Check sheet for the drawn part. Datum: minimum x, y, z corner. Units: mm. Coordinates: 2 decimals unless noted, no trailing zeros. Loops run counter-clockwise (first coordinate to the right, second up) from the corner with the lowest first, then second, coordinate; pieces in that order, holes last. Notation, with made-up numbers: (56.5, -26) -> (70.5, -26) arc R14 ccw to (70.5, -4) -> close; hole circle Ø8 at (73, 67.25). An arc over 180 degrees is marked (long way). Use CSV: the item, a comma, the result in double quotes. Start each with the question number.
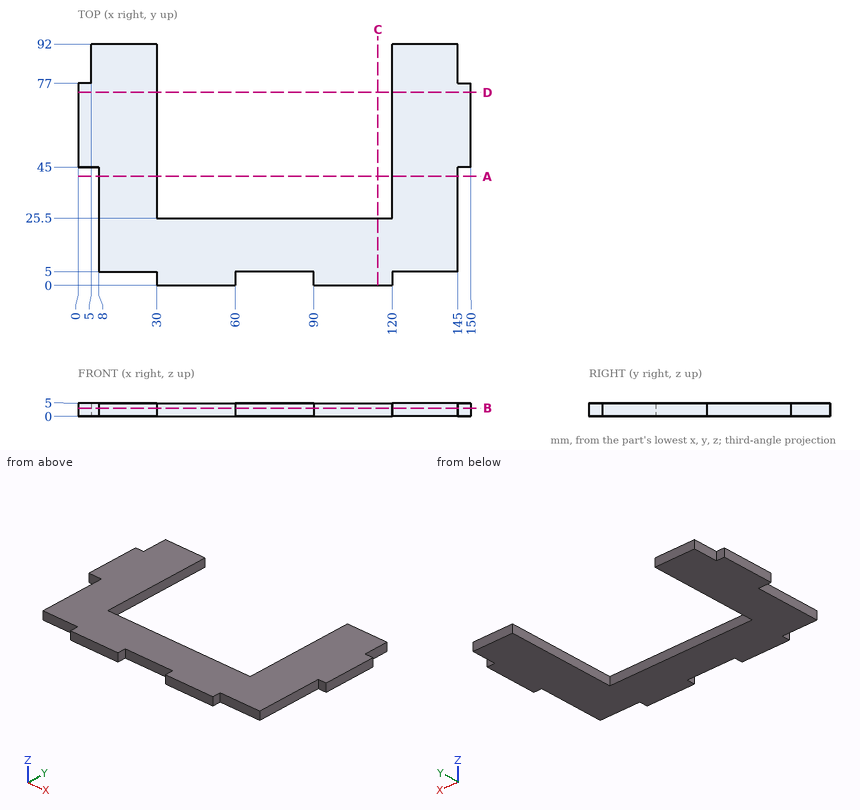
1. Cross-section at C-C, the plane x = 114.5. Record the boundary of the cut face in (y, z).
2. Cross-section at D-D, the plane y = 73.5. Record the boundary of the cut face in (x, z), plus the area to 3 significant figures.
3. Cross-section at A-A, the plane y = 41.5. Record the boundary of the cut face in (x, z).
4. Scan lines: line 1 (X direction, y = 29, z = 2.75); line 2 (X direction, y = 84.5, z = 4.55); line 3 (Y direction, x = 30.5, z = 2.9). Record each from-to range of solid material in increasing order.
5. Depth check by flat-ended pin: pin 1 (2.5 mm diameter, centred on x = 2, z = 1.5, fed in from -Y); pin 2 (2 mm diameter, centred on x = 123.5, z = 3, fed in from -Y); pin 3 (1.5 mm diameter, centred on y = 84.5, z = 1.5, fed in from -X). Enter the tip coordinate at first touch or a pass-through.
6. Cross-section at B-B, the plane z = 3.05. Record the boundary of the cut face in (x, y), plus the area to 4 significant figures.
Solution:
1,outline,"(0, 0) -> (25.5, 0) -> (25.5, 5) -> (0, 5) -> close"
2,outline,"(0, 0) -> (30, 0) -> (30, 5) -> (0, 5) -> close; (120, 0) -> (150, 0) -> (150, 5) -> (120, 5) -> close"
2,area,"300 mm2"
3,outline,"(8, 0) -> (30, 0) -> (30, 5) -> (8, 5) -> close; (120, 0) -> (145, 0) -> (145, 5) -> (120, 5) -> close"
4,line 1,"x = 8 to 30, 120 to 145"
4,line 2,"x = 5 to 30, 120 to 145"
4,line 3,"y = 0 to 25.5"
5,pin 1,"stops at y = 45"
5,pin 2,"stops at y = 5"
5,pin 3,"stops at x = 5"
6,outline,"(0, 45) -> (8, 45) -> (8, 5) -> (30, 5) -> (30, 0) -> (60, 0) -> (60, 5) -> (90, 5) -> (90, 0) -> (120, 0) -> (120, 5) -> (145, 5) -> (145, 45) -> (150, 45) -> (150, 77) -> (145, 77) -> (145, 92) -> (120, 92) -> (120, 25.5) -> (30, 25.5) -> (30, 92) -> (5, 92) -> (5, 77) -> (0, 77) -> close"
6,area,"6,695 mm2"
